from build123d import *

# Parameters (mm, degrees)
F1_DEPTH      = 150
F3_DEPTH      = 34.5108737383
F3_DEPTH_BACK = 34.5108737383


with BuildPart() as f1:
    # F0 (on Right) → F1 (new body)
    with BuildSketch(Plane.YZ):
        with BuildLine():
            Line((34.5098737383, 37.8046733585), (-34.5098737383, 37.8046733585))
            Line((-34.5098737383, 37.8046733585), (-31.0674993665, 9.7687839396))
            ThreePointArc((-31.0674993665, 9.7687839396), (-29.0879427459, 6.0062656753), (-25.1122224566, 4.5))
            Line((-25.1122224566, 4.5), (25.1122224566, 4.5))
            ThreePointArc((25.1122224566, 4.5), (29.0879427459, 6.0062656753), (31.0674993665, 9.7687839396))
            Line((31.0674993665, 9.7687839396), (34.5098737383, 37.8046733585))
        make_face()
    extrude(amount=F1_DEPTH)

    # F2 (on Front) → F3 (cut, two sides)
    with BuildSketch(Plane.XZ) as f3_sk:
        Polygon((4.0892996943, 4.5), (0, 37.8046733585), (0, 4.5), align=None)
        Polygon((150, 37.8046733585), (145.9107003057, 4.5), (150, 4.5), align=None)
    extrude(amount=-F3_DEPTH, mode=Mode.SUBTRACT)
    extrude(f3_sk.sketch, amount=F3_DEPTH_BACK, mode=Mode.SUBTRACT)


solid = f1.part
Source: CAD feature listing. Evaluate the final solid. Frame: model axes, mm. Give positions to 0.01 mm unless a question says otherwise; leave off trailing zeros. Write each loop counter-clockwise with the first axis right and the second up, starting at its lowest first coordinate (ties: lowest second). Pieces come first, ordered by that corner, then holes. Notation, with made-up numbers: (41.25, 43.25) -> (92.25, 43.25) arc R12 cw to (92.25, 47.25) -> close; hole circle Ø10 at (88, 45). An arc over 180 degrees is marked (long way). Return JSON: item names as keys, results as strings. Group by question number.
1. Material intervals for line 1 (X direction, y = -16, z = 15.5); line 2 (X direction, y = 13.5, z = 24) (3 decimals); line 3 (Y direction, x = 35, z = 18), sorted ascending. Write a range as from..to.
2. Pin query (flat end, axial travel): pin 1 Ø1 at (x, z) = (24, 24) entering from -Y; pin 2 Ø12 at (y, z) = (-24.5, 32) entering from +X; pin 3 Ø12 at (x, z) = (22, 20) entering from -Y. Return the tip coordinate at first contact, or that it passes through.
3. Section A-A, the plane x = 80. Output: boundary loops of the cut face in (y, z).
4. Section B-B, the plane y = -13. Output: boundary loops of the cut face in (x, z), then the cut area to 3 significant figures.
5. Section C-C, the plane z = 19. Output: boundary loops of the cut face in (x, y), then the cut area to 3 significant figures.
Determined:
{
 "1": {"line 1": "x = 2.74..147.26", "line 2": "x = 1.695..148.305", "line 3": "y = -32.08..32.08"},
 "2": {"pin 1": "stops at y = -32.88", "pin 2": "stops at x = 150", "pin 3": "stops at y = -33.06"},
 "3": {"outline": "(-34.51, 37.8) -> (-31.07, 9.77) arc R6 ccw to (-25.11, 4.5) -> (25.11, 4.5) arc R6 ccw to (31.07, 9.77) -> (34.51, 37.8) -> close"},
 "4": {"outline": "(0, 37.8) -> (4.09, 4.5) -> (145.91, 4.5) -> (150, 37.8) -> close", "area": "4,860 mm2"},
 "5": {"outline": "(2.31, -32.2) -> (147.69, -32.2) -> (147.69, 32.2) -> (2.31, 32.2) -> close", "area": "9,360 mm2"}
}
